The listing builds one solid part. Answer for the finished solid, in the listing's coordinates (mm). Give positions to 0.01 mm unless a question says otherwise; leave off trailing zeros. Loops run counter-clockwise (first coordinate to the right, second up) from the corner with the lowest first, then second, coordinate; pieces in that order, holes last. Notation, with made-up numbers: (31, 39.25) - (65, 39.25) arc R18 ccw to (65, 58.25) - close; hole circle Ø5 at (44.5, 58). An arc over 180 degrees is marked (long way). Write each question's results on one line, items separated by ' | '.
Autodesk Fusion 360 part; units mm, degrees
sketch "Sketch1" plane through (0, 0, 0) normal (0, 1, 0) x (1, 0, 0)
  line L0 (0, 0) -> (12, 0)
  line L1 (12, 0) -> (12, -12)
  line L2 (12, -12) -> (0, -12)
  line L3 (0, -12) -> (0, 0)
  circle A0 centre (6, -6) radius 3.75
  line L4 (6, 0) -> (6, -12) construction
  circle A1 centre (6, -6) radius 5
  line L5 (2, -12) -> (2, -9) construction
  line L6 (1, -12) -> (1, -6)
  line L7 (3, -10) -> (3, -12)
  arc A2 (7.5, -12) -> (4.5, -12) centre (6, -13.7) ccw
  dimension "d1" = 12
  dimension "d2" = 12
  dimension "d3" = 7.5
  dimension "d4" = 10
  dimension "d5" = 4
  dimension "d6" = 2
  dimension "d16" = 3
  dimension "d17" = 1.7
extrude "Extrude1" add sketch "Sketch1" against normal blind 1 contours L0 L1 L2 L3 A1 L6 L7 A2 | L2 A1 L6 L7 | A1
extrude "Extrude2" cut sketch "Sketch1" against normal blind 0.3 contours A1
extrude "Extrude3" cut sketch "Sketch1" against normal blind 0.3 contours L2 A1 L6 L7
ref_plane "WorkPlane1" through (6, -0.5, 6) normal (1, 0, 0) x (0, 0, 1)
mirror "Mirror1" about plane through (6, -0.5, 6) normal (1, 0, 0) of "Extrude3"
fillet "Fillet1" radius 6 2 edges at (0, -0.5, 0) (12, -0.5, 0)
fillet "Fillet2" radius 0.5 2 edges at (3, -0.15, 10) (9, -0.15, 10)
equation "d3 = ( 3.75 * 2 ) * 1 mm"
Item 1: A cutting plane is placed at C-C, the plane x = 6.5. Determine the outline of the cut face in (y, z).
Values found:
outline: (-1, 0.02) - (0, 0.02) - (0, 1.03) - (-0.3, 1.03) - (-0.3, 2.28) - (-1, 2.28) - close; (-1, 9.72) - (-0.3, 9.72) - (-0.3, 10.97) - (0, 10.97) - (0, 11.49) - (-1, 11.49) - close
Item 2: Flat-ended cylindrical pins translate along their axes: P1, Ø5, axis at x = 10.5, z = 9, coming from the +Y side; P2, Ø3, axis at x = 7, z = 6.5, coming from the +Y side. Find the tip coordinate at first contact, or state that the pin passes through.
Values found:
P1: stops at y = 0 | P2: passes through
Item 3: For a pull along X with two mould halves and no side action, classify faces 1 (the face through (6, -0.3, 10)), 2 (the face through (10.196, -0.507, 1.711)), 3 (the face through (6, -1, 10)) as released by +X, released by -X, zero draft, split by the parting line, or undercut.
Values found:
face 1: undercut | face 2: released by +X | face 3: zero draft
Item 4: Find the intervals of material crossed by line 1 along Z through (x, y) = (6, -0.6); line 2 along X through (y, z) = (-0.7, 6); line 3 along X through (y, z) = (-0.25, 8.5), in increasing order. Write a range as [from, to].
Values found:
line 1: z = [0, 2.25], [9.75, 11.43] | line 2: x = [0, 2.25], [9.75, 12] | line 3: x = [0, 1], [11, 12]
Item 5: A cutting plane is placed at D-D, the plane z = 2. Determine the outline of the cut face in (x, y).
Values found:
outline: (1.53, -1) - (10.47, -1) - (10.47, 0) - (9, 0) - (9, -0.3) - (3, -0.3) - (3, 0) - (1.53, 0) - close
Item 6: A cutting plane is placed at A-A, the plane z = 9. Determine the outline of the cut face in (x, y), plus the area to 3 significant figures.
Values found:
outline: (0, -1) - (3.75, -1) - (3.75, -0.3) - (1, -0.3) - (1, 0) - (0, 0) - close; (8.25, -1) - (12, -1) - (12, 0) - (11, 0) - (11, -0.3) - (8.25, -0.3) - close | area: 5.85 mm²
